Source: CAD feature listing. Evaluate the final solid. Frame: model axes, mm. Coordinates: 2 decimals unless noted, no trailing zeros. Order: outer loops, then holes, each group sorted by start corner. A loop starts at its lowest first (then second) coordinate and runs counter-clockwise, first axis right, second up.
```python
from build123d import *

# Parameters (mm, degrees)
F0_W     = 50
F0_H     = 75
F1_DEPTH = 50
F3_D     = 25


with BuildPart() as f1:
    # F0 (on Front) → F1 (new body, symmetric)
    with BuildSketch(Plane.XZ):
        with Locations((-11.862348, 35.03312)):
            Rectangle(F0_W, F0_H)
    extrude(amount=F1_DEPTH, both=True)

    # F3 (through all)
    with Locations(Plane.YZ.offset(13.137652)):
        with Locations((15.938677, 40.338628)):
            Hole(F3_D / 2)


solid = f1.part
```
1. Section query C-C on x = -26.5. Return loops of the section in (y, z).
Findings:
outline: (-50, -2.47) - (50, -2.47) - (50, 72.53) - (-50, 72.53) - close; hole circle Ø25 at (15.94, 40.34)
2. Ray query, line 1 (Z direction, x = -5.5, y = 19); line 2 (Z direction, x = -11.5, y = 8.5); line 3 (Y direction, x = 7.5, z = 38.5). Return the intervals inside material, ascending.
Findings:
line 1: z = -2.47 to 28.22, 52.46 to 72.53
line 2: z = -2.47 to 30.29, 50.38 to 72.53
line 3: y = -50 to 3.57, 28.3 to 50
3. Section query B-B on z = 30.5. Return loops of the section in (x, y).
Findings:
outline: (-36.86, -50) - (13.14, -50) - (13.14, 8.23) - (-36.86, 8.23) - close; (-36.86, 23.65) - (13.14, 23.65) - (13.14, 50) - (-36.86, 50) - close
4. Section query A-A on y = 18.5. Return loops of the section in (x, z).
Findings:
outline: (-36.86, -2.47) - (13.14, -2.47) - (13.14, 28.1) - (-36.86, 28.1) - close; (-36.86, 52.57) - (13.14, 52.57) - (13.14, 72.53) - (-36.86, 72.53) - close
5. Draft query along Y for faces 1 (the face through (-12.212, 4.392, 35.551)), 2 (the face through (13.138, -1, 35)), 3 (the face through (-12, -50, 36)). Return one class per face: released by +Y, released by -Y, zero draft, split by the parting line, or undercut.
Findings:
face 1: undercut
face 2: zero draft
face 3: released by -Y
6. Pin query (flat end, axial travel): P1, Ø20, axis at y = 15.94, z = 40.34, coming from the +X side. Return the tip coordinate at first contact, or that it passes through.
Findings:
P1: passes through
